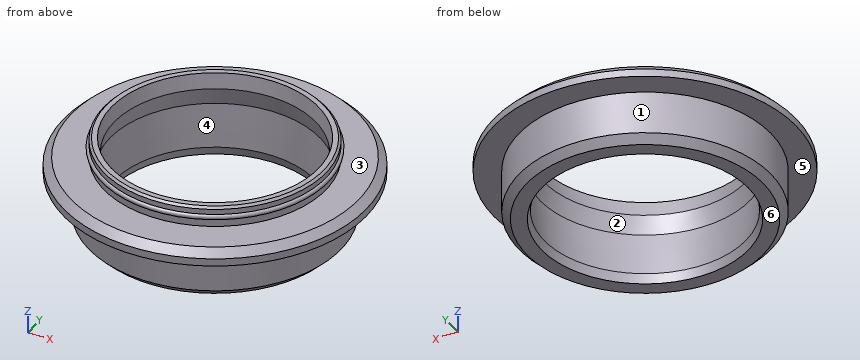
```python
from build123d import *


with BuildPart() as f1:
    # F0 (on Front) → F1 (revolve)
    with BuildSketch(Plane.XZ):
        with BuildLine():
            Line((-23.5, 0), (-20.53616, 0))
            Line((-20.53616, 0), (-20, 1.783461))
            Line((-20, 1.783461), (-20.832418, 10.402767))
            Line((-20.832418, 10.402767), (-20, 13.996847))
            Line((-20, 13.996847), (-20.519255, 17))
            Line((-20.519255, 17), (-21.558487, 17))
            Line((-21.558487, 17), (-22, 16.558487))
            Line((-22, 16.558487), (-22, 15.5))
            ThreePointArc((-22, 15.5), (-22.5, 15), (-22, 14.5))
            Line((-22, 14.5), (-22, 13))
            Line((-22, 13), (-28.5, 13))
            Line((-28.5, 13), (-30, 11.5))
            Line((-30, 11.5), (-30, 10))
            Line((-30, 10), (-25, 10))
            Line((-25, 10), (-25, 1.5))
            Line((-25, 1.5), (-23.5, 0))
        make_face()
    revolve(axis=Axis((0, 0, 21.225085), (0, 0, 1)))


solid = f1.part
```
Here's how the part is built. I have some questions about the finished solid (model axes, mm). Face numbers are marked on the shaded views. A direction names the side the tool comes from. Coordinates: 2 decimals unless noted, no trailing zeros. Order: outer loops, then holes, each group sorted by start corner. A loop starts at its lowest first (then second) coordinate and runs counter-clockwise, first axis right, second up.
1) Which directions (+Z, -Z, +X, -X, +Y, -Y) give clear straight access to the entire face, cutting with the end or side of a thin tool? Please do the marked faces 4, 5 and 6.
2) Imagine slicing it at C-C on z = 6.75. List the corners of the cut face in (x, y) for me.
3) Will these pins go through, and if not, where does the flat tip stop? pin 1 (2 mm diameter, centred on y = 10.5, z = 8, fed in from -X); pin 2 (1 mm diameter, centred on y = 13, z = 15, fed in from +X); pin 3 (2 mm diameter, centred on x = -6, z = 12.5, fed in from -Y).
4) I need wall thicknesses on line 1 (X direction, y = 7, z = 1.5); line 2 (Y direction, x = -14.5, z = 8.5); line 3 (X direction, y = 10.5, z = 5). Which ranges of each line are inside material? Lowest first, please.
5) We'd pull the mould along Y, two halves only. Please class the marked faces 1, 2 and 3: +Y half, -Y half, draft (parallel to the pull), parting line (faces both ways), or undercut.
Response values:
1. face 4: none
1. face 5: -Z
1. face 6: -Z, +X, -X, +Y, -Y
2. outline: circle Ø50 at (0, 0); hole circle Ø40.96 at (0, 0)
3. pin 1: stops at x = -23.12
3. pin 2: stops at x = 18.71
3. pin 3: stops at y = -29.41
4. line 1: x = -24 to -18.83, 18.83 to 24
4. line 2: y = -20.37 to -14.7, 14.7 to 20.37
4. line 3: x = -22.69 to -17.39, 17.39 to 22.69
5. face 1: parting line
5. face 2: undercut
5. face 3: draft
